```python
from build123d import *

# Parameters (mm, degrees)
SKETCH1_R           = 30
BOSS_EXTRUDE1_DEPTH = 8
SKETCH2_R           = 30
SKETCH2_R_2         = 28
BOSS_EXTRUDE2_DEPTH = 17
CUT_EXTRUDE1_DEPTH  = 39
CIRPATTERN1_COUNT   = 2
CIRPATTERN1_ANGLE   = 180
CUT_EXTRUDE2_DEPTH  = 4
SKETCH4_4_R         = 1.5
CUT_EXTRUDE3_DEPTH  = 20


with BuildPart() as part:
    # Sketch1 → Boss-Extrude1 (new body)
    with BuildSketch(Plane.XY):
        Circle(SKETCH1_R)
    extrude(amount=BOSS_EXTRUDE1_DEPTH)

    # Sketch2 → Boss-Extrude2 (add)
    with BuildSketch(Plane.XY.offset(8)):
        Circle(SKETCH2_R)
        Circle(SKETCH2_R_2, mode=Mode.SUBTRACT)
    extrude(amount=BOSS_EXTRUDE2_DEPTH)

    # Sketch3 → Cut-Extrude1 (cut)
    with BuildSketch(Plane(origin=(0, 0, 0), x_dir=(0, 0, -1), z_dir=(1, 0, 0))):
        with BuildLine():
            Line((-25, 3), (-20, 3))
            Line((-20, 3), (-14, 3))
            Line((-14, 3), (-14, -9))
            ThreePointArc((-14, -9), (-14.878679656, -11.121320344), (-17, -12))
            Line((-17, -12), (-20, -12))
            ThreePointArc((-20, -12), (-23, -9), (-20, -6))
            Line((-20, -6), (-20, -3))
            Line((-20, -3), (-25, -3))
            Line((-25, -3), (-25, 3))
        make_face()
    cut_extrude1 = extrude(amount=-CUT_EXTRUDE1_DEPTH, mode=Mode.SUBTRACT)

    # CirPattern1: Cut-Extrude1 ×2 about axis
    cirpattern1_axis = Axis((0, 0, 8), (0, 0, 1))
    for i in range(1, CIRPATTERN1_COUNT):
        add(cut_extrude1.rotate(cirpattern1_axis, i * CIRPATTERN1_ANGLE / (CIRPATTERN1_COUNT - 1)), mode=Mode.SUBTRACT)

    # Sketch4 → Cut-Extrude2 (cut)
    with BuildSketch(Plane(origin=(0, 0, 0), x_dir=(-1, 0, 0), z_dir=(0, 0, -1))):
        with BuildLine():
            Line((-3.375, 24), (-3.375, 12.024350294))
            ThreePointArc((-3.375, 12.024350294), (-4.02628005, 8.050346325), (-5.911981132, 4.49211577))
            ThreePointArc((-5.911981132, 4.49211577), (0, -7.425), (5.911981132, 4.49211577))
            ThreePointArc((5.911981132, 4.49211577), (4.02628005, 8.050346325), (3.375, 12.024350294))
            Line((3.375, 12.024350294), (3.375, 24))
            ThreePointArc((3.375, 24), (0, 27.375), (-3.375, 24))
        make_face()
    extrude(amount=-CUT_EXTRUDE2_DEPTH, mode=Mode.SUBTRACT)

    # Sketch4<4> → Cut-Extrude3 (cut)
    with BuildSketch(Plane(origin=(0, 0, 0), x_dir=(-1, 0, 0), z_dir=(0, 0, -1))):
        with Locations((0, 24)):
            Circle(SKETCH4_4_R)
        with Locations((0, 20)):
            Circle(SKETCH4_4_R)
    extrude(amount=-CUT_EXTRUDE3_DEPTH, mode=Mode.SUBTRACT)


solid = part.part
```
Source: CAD feature listing. Evaluate the final solid. Frame: model axes, mm. A direction names the side the tool comes from. Coordinates: 2 decimals unless noted, no trailing zeros. Write each loop counter-clockwise with the first axis right and the second up, starting at its lowest first coordinate (ties: lowest second). Pieces come first, ordered by that corner, then holes. Notation, with made-up numbers: (-27, 64) - (23, 64) arc R17 ccw to (23, 89) - close; hole circle Ø9 at (18, -16). An arc over 180 degrees is marked (long way). Answer as a JSON object with one key per item and string values.
Q1. Section query C-C, the plane z = 15.5. Output: boundary loops of the cut face in (x, y).
Ans:
{"outline": "(-29.85, 3) - (-27.84, 3) arc R28 cw to (25.48, 11.6) - (27.67, 11.6) arc R30 ccw to start; (-27.67, -11.6) arc R30 ccw to (29.85, -3) - (27.84, -3) arc R28 cw to (-25.48, -11.6) - close"}
Q2. Section query B-B, the plane y = 0. Output: boundary loops of the cut face in (x, z) (3 decimals), plus the area to 3 significant figures.
Ans:
{"outline": "(-30, 0) - (-7.425, 0) - (-7.425, 4) - (7.425, 4) - (7.425, 0) - (30, 0) - (30, 14) - (28, 14) - (28, 8) - (-28, 8) - (-28, 14) - (-30, 14) - close", "area": "445 mm2"}
Q3. Set-up query: faces 1 (the flat face through (26, 12, 18)), 2 (the flat face through (-29, -3, 22)), 3 (the cylindrical face through (4.01, 8.1, 1.97)). Return all of +Z, -Z, +X, -X, +Y, -Y with unobstructed straight access to the full face (end or side cutting, diameter ignored); none if empty.
Ans:
{"face 1": "+X", "face 2": "+Z, +X, -X", "face 3": "-Z"}
Q4. Material intervals for line 1 (Y direction, x = 0, z = 6.1); line 2 (Y direction, x = 0, z = 20.5); line 3 (Y direction, x = 0, z = 1.85) (3 decimals), sorted ascending. Write a range as [from, to].
Ans:
{"line 1": "y = [-30, 18.5], [21.5, 22.5], [25.5, 30]", "line 2": "y = [-30, -28], [28, 30]", "line 3": "y = [-30, -7.425], [27.375, 30]"}
Q5. Section query D-D, the plane z = 6. Output: boundary loops of the cut face in (x, y).
Ans:
{"outline": "circle Ø60 at (0, 0); hole circle Ø3 at (0, 20); hole circle Ø3 at (0, 24)"}
Q6. Draft query along Z for faces 4 (the flat face through (-29, -5, 20)), 5 (the cylindrical face through (0.23, -7.42, 1.97)), 6 (the flat face through (0, 6, 4)). Return one class per face: released by +Z, released by -Z, zero draft, split by the parting line, or undercut.
Ans:
{"face 4": "undercut", "face 5": "zero draft", "face 6": "released by -Z"}
Q7. First-contact query: pin 1 Ø4.5 at (y, z) = (17.5, 1.5) entering from +X; pin 2 Ø2 at (x, z) = (-19.5, 17) entering from +Y; pin 3 Ø2.5 at (x, y) = (0, 24) entering from +Z; pin 4 Ø5 at (x, y) = (19, -2) entering from +Z. Flat tips, straight axial feed; report the tip coordinate or a pass-through.
Ans:
{"pin 1": "stops at x = 25.83", "pin 2": "stops at y = 23.62", "pin 3": "passes through", "pin 4": "stops at z = 8"}
Q8. Section query A-A, the plane x = 0. Output: boundary loops of the cut face in (y, z) (3 decimals).
Ans:
{"outline": "(-30, 0) - (-7.425, 0) - (-7.425, 4) - (18.5, 4) - (18.5, 8) - (-28, 8) - (-28, 25) - (-30, 25) - close; (21.5, 4) - (22.5, 4) - (22.5, 8) - (21.5, 8) - close; (25.5, 4) - (27.375, 4) - (27.375, 0) - (30, 0) - (30, 25) - (28, 25) - (28, 8) - (25.5, 8) - close"}
